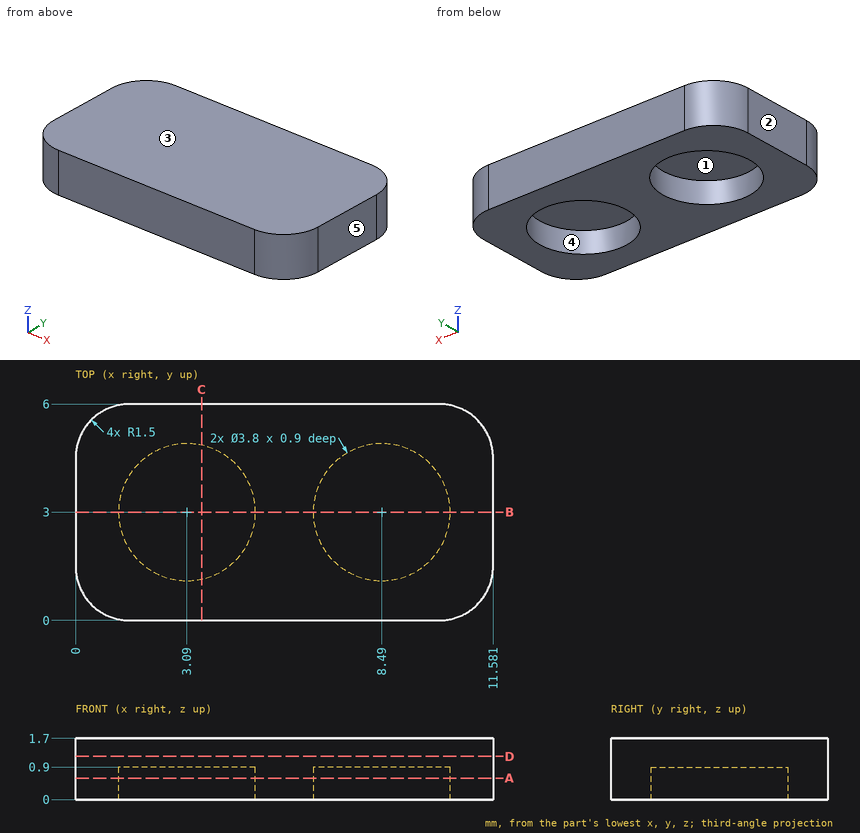
Part print with two shaded views. Sizes in mm from the minimum x, y, z corner. A direction names the side the tool comes from. Give positions to 0.01 mm unless a question says otherwise; leave off trailing zeros. Loops run counter-clockwise (first coordinate to the right, second up) from the corner with the lowest first, then second, coordinate; pieces in that order, holes last. Notation, with made-up numbers: (50, -1.5) - (72, -1.5) arc R26 cw to (72, 13.5) - close; hole circle Ø8 at (-16, -25). An arc over 180 degrees is marked (long way). Put each result on its own line as item: value.
Q1. Flat gauge pin, fed straight in: pin 1 (1.1 mm diameter, centred on x = 3.5, y = 3.5, fed in from -Z). Where does the tip first touch, or does it go through?
Filled in:
pin 1: stops at z = 0.9
Q2. Mould opens along X. For the marked faces 1, 2 and 3 say: pulls with the +X half, pulls with the -X half, needs draft (parallel to the pull), parting line crosses it, or undercut.
Filled in:
face 1: undercut
face 2: pulls with the -X half
face 3: needs draft
Q3. Probe line 1 along X through (y, z) = (3, 0.6); line 2 along X through (y, z) = (1.3, 0.2) (1 decimal); line 3 along Y through (x, z) = (8.5, 0.55). List the from-to ranges inside material, lowest first.
Filled in:
line 1: x = 0 to 1.19, 4.99 to 6.59, 10.39 to 11.58
line 2: x = 0 to 2.2, 3.9 to 7.6, 9.3 to 11.6
line 3: y = 0 to 1.1, 4.9 to 6
Q4. Tool access for the marked faces 4 and 5: list every direction of +Z, -Z, +X, -X, +Y, -Y with a clear straight run to the whole face (end or side of a thin tool).
Filled in:
face 4: -Z
face 5: +Z, -Z, +X, +Y, -Y
Q5. Slice it at B-B (y = 3). Give the cut face in (x, z).
Filled in:
outline: (0, 0) - (1.19, 0) - (1.19, 0.9) - (4.99, 0.9) - (4.99, 0) - (6.59, 0) - (6.59, 0.9) - (10.39, 0.9) - (10.39, 0) - (11.58, 0) - (11.58, 1.7) - (0, 1.7) - close
Q6. Slice it at A-A (z = 0.6). Give the cut face in (x, y).
Filled in:
outline: (0, 1.5) arc R1.5 ccw to (1.5, 0) - (10.08, 0) arc R1.5 ccw to (11.58, 1.5) - (11.58, 4.5) arc R1.5 ccw to (10.08, 6) - (1.5, 6) arc R1.5 ccw to (0, 4.5) - close; hole circle Ø3.8 at (3.09, 3); hole circle Ø3.8 at (8.49, 3)
Q7. Slice it at D-D (z = 1.2). Give the cut face in (x, y).
Filled in:
outline: (0, 1.5) arc R1.5 ccw to (1.5, 0) - (10.08, 0) arc R1.5 ccw to (11.58, 1.5) - (11.58, 4.5) arc R1.5 ccw to (10.08, 6) - (1.5, 6) arc R1.5 ccw to (0, 4.5) - close
Q8. Slice it at C-C (x = 3.5). Give the cut face in (y, z) (1 decimal).
Filled in:
outline: (0, 0) - (1.1, 0) - (1.1, 0.9) - (4.9, 0.9) - (4.9, 0) - (6, 0) - (6, 1.7) - (0, 1.7) - close
